Geometry: final body of the model. Coordinates: model frame, mm. Face numbers are marked on the shaded views. A direction names the side the tool comes from. Coordinates: 2 decimals unless noted, no trailing zeros. Loops run counter-clockwise (first coordinate to the right, second up) from the corner with the lowest first, then second, coordinate; pieces in that order, holes last. Notation, with made-up numbers: (73, 88) -> (127, 88) arc R27 ccw to (127, 112) -> close; hole circle Ø6 at (-4.5, 59.25). An arc over 180 degrees is marked (long way). One line per item, written item: value. Start each with the question number.
Item 1: Section query C-C on y = -6.5. Return loops of the section in (x, z), then the cut area to 3 significant figures.
Item 2: Set-up query: the marked faces 4 and 5. Return all of +Z, -Z, +X, -X, +Y, -Y with unobstructed straight access to the full face (end or side cutting, diameter ignored); none if empty.
Item 3: Ray query, probe 1 along Y at (x, z) = (4.5, 1.6); probe 2 along X at (y, z) = (2.5, 6.5); probe 3 along Z at (x, y) = (1, -0.75). Return the intervals inside material, ascending. Write a range as from..to.
Item 4: Mould query, pull axis X, two halves, no side actions, for the marked faces 1, 2 and 3. Classes: +X half, -X half, draft (parallel to the pull), parting line (faces both ways), or undercut.
Item 5: Section query A-A on z = 40. Return loops of the section in (x, y).
Item 6: Section query D-D on z = 8. Return loops of the section in (x, y), then the cut area to 3 significant figures.
Item 7: Section query B-B on x = -4.5. Return loops of the section in (y, z), then the cut area to 3 significant figures.
Item 8: Contact query for a flat-ended pin moving along its axis: pin 1 Ø4 at (x, y) = (-4.5, 6.5) entering from +Z. Output: stop coordinate, or through.
from build123d import *

# Parameters (mm, degrees)
SKETCH_1_W          = 26
SKETCH_1_H          = 20
EXTRUDE_1_DEPTH     = 4
SKETCH_2_W          = 4
SKETCH_2_H          = 20
EXTRUDE_2_DEPTH     = 40
SKETCH_3_R          = 1.5
CUT_EXTRUDE_1_DEPTH = 30
CUT_EXTRUDE_2_DEPTH = 53.076866265
FILLET_1_R          = 2


with BuildPart() as part:
    # 草图1 → 凸台-拉伸1 (new body)
    with BuildSketch(Plane.XY):
        Rectangle(SKETCH_1_W, SKETCH_1_H)
    extrude(amount=EXTRUDE_1_DEPTH)

    # 草图2 → 凸台-拉伸2 (add)
    with BuildSketch(Plane.XY.offset(4)):
        with Locations((-11, 0)):
            Rectangle(SKETCH_2_W, SKETCH_2_H)
        with Locations((11, 0)):
            Rectangle(SKETCH_2_W, SKETCH_2_H)
    extrude(amount=EXTRUDE_2_DEPTH)

    # 草图3 → 切除-拉伸1 (cut)
    with BuildSketch(Plane.XY.offset(4)):
        with Locations((-4.5, 6.5)):
            Circle(SKETCH_3_R)
        with Locations((4.5, 6.5)):
            Circle(SKETCH_3_R)
        with Locations((4.5, -6.5)):
            Circle(SKETCH_3_R)
        with Locations((-4.5, -6.5)):
            Circle(SKETCH_3_R)
    extrude(amount=-CUT_EXTRUDE_1_DEPTH, mode=Mode.SUBTRACT)

    # 草图4 → 切除-拉伸2 (cut, through all)
    with BuildSketch(Plane(origin=(13, 0, 0), x_dir=(0, 0, -1), z_dir=(1, 0, 0))):
        Polygon((-44, -7), (-4, 10), (-44, 10), align=None)
    extrude(amount=-CUT_EXTRUDE_2_DEPTH, mode=Mode.SUBTRACT)

    # 圆角1
    fillet_1_edges = [part.edges().sort_by_distance(p)[0] for p in [
        (-9, 0, 4),
        (9, 0, 4),
    ]]
    fillet(fillet_1_edges, radius=FILLET_1_R)


solid = part.part
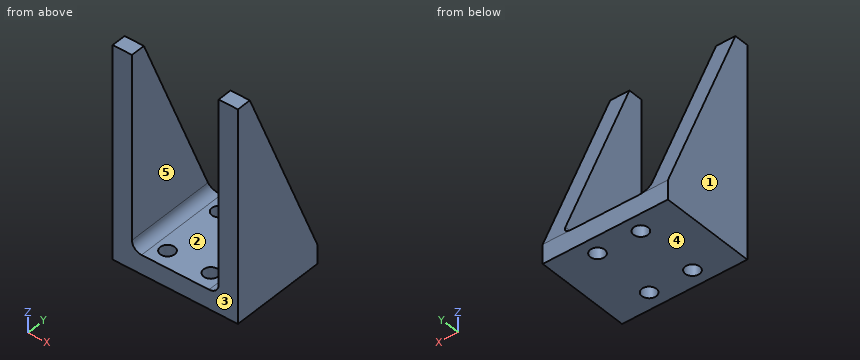
Reply:
1. outline: (-13, 0) -> (-6, 0) -> (-6, 4) -> (-7, 4) arc R2 cw to (-9, 6) -> (-9, 42.82) -> (-13, 42.82) -> close; (-3, 0) -> (3, 0) -> (3, 4) -> (-3, 4) -> close; (6, 0) -> (13, 0) -> (13, 42.82) -> (9, 42.82) -> (9, 6) arc R2 cw to (7, 4) -> (6, 4) -> close
1. area: 392 mm²
2. face 4: -Z, +X, -X, +Y, -Y
2. face 5: +Z, +Y, -Y
3. probe 1: y = -10..-8, -5..5, 8..10
3. probe 2: x = -13..-9, 9..13
3. probe 3: z = 0..4
4. face 1: -X half
4. face 2: undercut
4. face 3: draft
5. outline: (-13, -10) -> (-9, -10) -> (-9, -5.3) -> (-13, -5.3) -> close; (9, -10) -> (13, -10) -> (13, -5.3) -> (9, -5.3) -> close
6. outline: (-13, -10) -> (-9, -10) -> (-9, 8.3) -> (-13, 8.3) -> close; (9, -10) -> (13, -10) -> (13, 8.3) -> (9, 8.3) -> close
6. area: 146 mm²
7. outline: (-10, 0) -> (-8, 0) -> (-8, 4) -> (-10, 4) -> close; (-5, 0) -> (5, 0) -> (5, 4) -> (-5, 4) -> close; (8, 0) -> (10, 0) -> (10, 4) -> (8, 4) -> close
7. area: 56.0 mm²
8. pin 1: stops at z = 4
